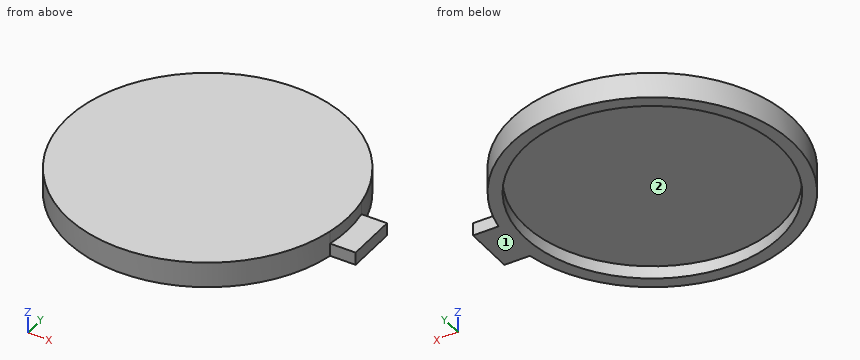
from build123d import *

# Parameters (mm, degrees)
SKETCH_1_R          = 55
SKETCH_1_R_2        = 50
EXTRUDE_1_DEPTH     = 5
SKETCH_3_R          = 55
EXTRUDE_2_DEPTH     = 5
SKETCH_5_W          = 10
SKETCH_5_H          = 20
EXTRUDE_3_DEPTH     = 10
CUT_EXTRUDE_START   = -5
CUT_EXTRUDE_1_DEPTH = 5


with BuildPart() as part:
    # 스케치1 → 보스-돌출1 (new body)
    with BuildSketch(Plane.XY):
        Circle(SKETCH_1_R)
        Circle(SKETCH_1_R_2, mode=Mode.SUBTRACT)
    extrude(amount=EXTRUDE_1_DEPTH)

    # 스케치3 → 보스-돌출2 (add)
    with BuildSketch(Plane.XY.offset(5)):
        Circle(SKETCH_3_R)
    extrude(amount=EXTRUDE_2_DEPTH)

    # 스케치5 → 보스-돌출3 (add)
    with BuildSketch(Plane.XY):
        with Locations((59.083269132, 0)):
            Rectangle(SKETCH_5_W, SKETCH_5_H)
    extrude(amount=EXTRUDE_3_DEPTH)

    # 스케치6 → 컷-돌출1 (cut)
    with BuildSketch(Plane.XY.offset(10).offset(CUT_EXTRUDE_START)):
        with BuildLine():
            Line((54.083269132, 10), (64.083269132, 10))
            Line((64.083269132, 10), (64.083269132, -10))
            Line((64.083269132, -10), (54.083269132, -10))
            ThreePointArc((54.083269132, -10), (55, 0), (54.083269132, 10))
        make_face()
    extrude(amount=CUT_EXTRUDE_1_DEPTH, mode=Mode.SUBTRACT)


solid = part.part
Build history of the part. All positions in model axes, mm. Face numbers are marked on the shaded views. Give positions to 0.01 mm unless a question says otherwise; leave off trailing zeros. Write each loop counter-clockwise with the first axis right and the second up, starting at its lowest first coordinate (ties: lowest second). Pieces come first, ordered by that corner, then holes. Notation, with made-up numbers: (6.5, -37) - (41.5, -37) arc R31 cw to (41.5, -12) - close; hole circle Ø9 at (64, -15.75). An arc over 180 degrees is marked (long way). Use one line per item in the form item = value. Start each with the question number.
1. Band-saw the part on C-C on x = -38. Write the cut outline in (y, z), plus the area to 3 significant figures.
2. Band-saw the part on B-B on y = 0. Write the cut outline in (x, z), plus the area to 3 significant figures.
3. Two-plate mould, pull along X, no slides. Class the marked faces 1 and 2: released by +X, released by -X, zero draft, split by the parting line, or undercut.
4. Band-saw the part on D-D on x = 0. Write the cut outline in (y, z), plus the area to 3 significant figures.
5. Drop flat-ended pins along their axis: pin 1 Ø1.5 at (y, z) = (-33.5, 6.5) entering from +X; pin 2 Ø3 at (x, y) = (58, 5) entering from +Z; pin 3 Ø2 at (x, y) = (4.5, 32) entering from -Z. Give the stop position or say it passes through.
6. Probe line 1 (Y direction, x = 0, z = 1.6); line 2 (Z direction, x = 24, y = -19.5); line 3 (Y direction, x = -41, z = 0.5). List the from-to ranges inside material, lowest first. Write a range as [from, to].
7. Band-saw the part on A-A on z = 3. Write the cut outline in (x, y).
Conclusion:
q1.outline = (-39.76, 0) - (-32.5, 0) - (-32.5, 5) - (32.5, 5) - (32.5, 0) - (39.76, 0) - (39.76, 10) - (-39.76, 10) - close
q1.area = 470 mm²
q2.outline = (-55, 0) - (-50, 0) - (-50, 5) - (50, 5) - (50, 0) - (64.08, 0) - (64.08, 5) - (55, 5) - (55, 10) - (-55, 10) - close
q2.area = 645 mm²
q3.face_1 = zero draft
q3.face_2 = undercut
q4.outline = (-55, 0) - (-50, 0) - (-50, 5) - (50, 5) - (50, 0) - (55, 0) - (55, 10) - (-55, 10) - close
q4.area = 600 mm²
q5.pin_1 = 44.19
q5.pin_2 = 5
q5.pin_3 = 5
q6.line_1 = [-55, -50], [50, 55]
q6.line_2 = [5, 10]
q6.line_3 = [-36.66, -28.62], [28.62, 36.66]
q7.outline = (54.08, -10) - (64.08, -10) - (64.08, 10) - (54.08, 10) arc R55 ccw (long way) to start; hole circle Ø100 at (0, 0)
